from build123d import *

# Parameters (mm, degrees)
RUNROUTE_R               = 44.45
RUNROUTE_R_2             = 38.9128
BOSS_EXTRUDE1_DEPTH      = 48.41875
BOSS_EXTRUDE1_DEPTH_BACK = 43.65625
OUTLETROUTE_R            = 19.05
OUTLETROUTE_R_2          = 15.0876
RUNROUTE_2_R             = 38.9128
CUT_EXTRUDE1_DEPTH       = 49.4187501
CUT_EXTRUDE1_DEPTH_BACK  = 51.349153098


with BuildPart() as part:
    # RunRoute → Boss-Extrude1 (new body, two sides)
    with BuildSketch(Plane.XY) as boss_extrude1_sk:
        Circle(RUNROUTE_R)
        Circle(RUNROUTE_R_2, mode=Mode.SUBTRACT)
    extrude(amount=BOSS_EXTRUDE1_DEPTH)
    extrude(boss_extrude1_sk.sketch, amount=-BOSS_EXTRUDE1_DEPTH_BACK)

    # Sweep1: sweep along a path in Sketch2
    with BuildLine(Plane(origin=(0, 0, 0), x_dir=(0, 0, -1), z_dir=(1, 0, 0))) as sweep1_path:
        ThreePointArc((-1.330135383, 63.5), (11.421089133, 24.848331737), (43.65625, 0))
    # OutletRoute → Sweep1 (sweep)
    with BuildSketch(Plane(origin=(0, 63.5, 1.330135383), x_dir=(1, 0, 0), z_dir=(0, 0.999780683, 0.02094242))):
        Circle(OUTLETROUTE_R)
        Circle(OUTLETROUTE_R_2, mode=Mode.SUBTRACT)
    sweep(path=sweep1_path.line)

    # RunRoute<2> → Cut-Extrude1 (cut, two sides)
    with BuildSketch(Plane.XY) as cut_extrude1_sk:
        Circle(RUNROUTE_2_R)
    extrude(amount=CUT_EXTRUDE1_DEPTH, mode=Mode.SUBTRACT)
    extrude(cut_extrude1_sk.sketch, amount=-CUT_EXTRUDE1_DEPTH_BACK, mode=Mode.SUBTRACT)

    # Sketch3 → Revolve1 (revolve)
    with BuildSketch(Plane(origin=(0, 0, 0), x_dir=(0, 0, -1), z_dir=(1, 0, 0))):
        Polygon((13.754155657, 63.815970854), (17.715686637, 63.898953099), (17.350245598, 81.344926069), (21.311776579, 81.427908314), (21.680489514, 63.825736638), (17.954867586, 59.940694015), (13.837137901, 59.854439874), align=None)
    revolve(axis=Axis((0, 63.5, 1.330135383), (0, 0.999780683, 0.02094242)))

    # Sketch3<5> → Revolve2 (revolve)
    with BuildSketch(Plane(origin=(0, 0, 0), x_dir=(0, 0, -1), z_dir=(1, 0, 0))):
        Polygon((-48.41875, -38.9128), (-48.41875, -44.45), (-86.51875, -44.45), (-86.51875, -49.9872), (-42.88155, -49.9872), (-37.34435, -44.45), (-37.34435, -38.9128), align=None)
        Polygon((43.65625, -38.9128), (43.65625, -44.45), (81.75625, -44.45), (81.75625, -49.9872), (38.11905, -49.9872), (32.58185, -44.45), (32.58185, -38.9128), align=None)
    revolve(axis=Axis((0, 0, 48.41875), (0, 0, 1)))


solid = part.part
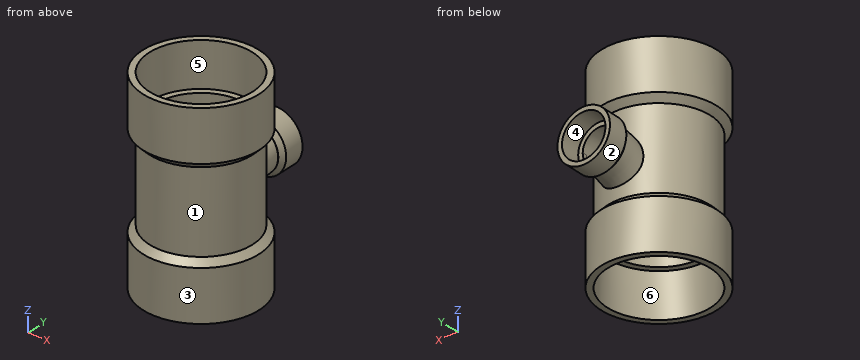
Design review of the part built by this model. Coordinates are the model's own, in mm. Face numbers are marked on the shaded views. A direction names the side the tool comes from. Round coordinates to 2 decimals unless told otherwise and drop trailing zeros. Write each loop counter-clockwise with the first axis right and the second up, starting at its lowest first coordinate (ties: lowest second). Pieces come first, ordered by that corner, then holes. Notation, with made-up numbers: (41.25, -40) -> (70.25, -40) arc R24 ccw to (70.25, -4) -> close; hole circle Ø8 at (56.25, -22). An arc over 180 degrees is marked (long way). One line per question, with ' | ' between items.
(1) Draft analysis for pull direction Z (two halves, no side actions). For the marked faces 1, 2 and 3, state which applies: released by +Z, released by -Z, zero draft, split by the parting line, or undercut.
Result sheet:
face 1: undercut | face 2: split by the parting line | face 3: zero draft
(2) Take a section at B-B, the plane z = 53. State the section outline as (x, y) points.
Result sheet:
outline: circle Ø99.97 at (0, 0); hole circle Ø88.9 at (0, 0)
(3) Wall thickness on line 1 (Y direction, x = 0, z = -10.5); line 2 (X direction, y = 0, z = 64.5); line 3 (Z direction, x = -12, y = 54): over which ranges is each line inside the solid? List them lowest first. Write a range as [from, to].
Result sheet:
line 1: [-44.45, -38.91], [38.91, 44.45] | line 2: [-49.99, -44.45], [44.45, 49.99] | line 3: [-14.56, -8.8], [9.72, 15.43]
(4) Take a section at C-C, the plane z = 27.5. State the section outline as (x, y) points, and give its area (3 significant figures).
Result sheet:
outline: circle Ø88.9 at (0, 0); hole circle Ø77.83 at (0, 0) | area: 1,450 mm2
(5) Take a section at A-A, the plane y = 0. State the section outline as (x, z) points, and give its area (3 significant figures).
Result sheet:
outline: (-49.99, -81.76) -> (-44.45, -81.76) -> (-44.45, -43.66) -> (-38.91, -43.66) -> (-38.91, 48.42) -> (-44.45, 48.42) -> (-44.45, 86.52) -> (-49.99, 86.52) -> (-49.99, 42.88) -> (-44.45, 37.34) -> (-44.45, -32.58) -> (-49.99, -38.12) -> close; (38.91, -43.66) -> (44.45, -43.66) -> (44.45, -81.76) -> (49.99, -81.76) -> (49.99, -38.12) -> (44.45, -32.58) -> (44.45, 37.34) -> (49.99, 42.88) -> (49.99, 86.52) -> (44.45, 86.52) -> (44.45, 48.42) -> (38.91, 48.42) -> close | area: 2,050 mm2
(6) Insertion check: P1, Ø4, axis at y = -1, z = 68, coming from the -X side; P2, Ø10, axis at y = -18, z = -15, coming from the -X side; P3, Ø2, axis at y = 30, z = 53, coming from the +X side. Each pin has a flat end and moves straight along its axis. Give the tip position at first contact, or say it passes through.
Result sheet:
P1: x = -49.99 | P2: x = -42.51 | P3: x = 40.72
(7) Machinability: for the marked faces 4, 5 and 6, which of the approach directions +Z, -Z, +X, -X, +Y, -Y give a long, thin tool a straight path to every point of the face, cutting with its end or side? Answer none if there is none.
Result sheet:
face 4: none | face 5: +Z | face 6: -Z
